from build123d import *

# Parameters (mm, degrees)
F0_R     = 4.1
F0_R_2   = 3.1
F1_DEPTH = 7
F2_SIZE  = 2


with BuildPart() as f1:
    # F0 (on Top) → F1 (new body)
    with BuildSketch(Plane.XY):
        with BuildLine():
            ThreePointArc((67.5, 27.5), (66.035534, 31.035534), (62.5, 32.5))
            Line((62.5, 32.5), (-62.5, 32.5))
            ThreePointArc((-62.5, 32.5), (-66.035534, 31.035534), (-67.5, 27.5))
            Line((-67.5, 27.5), (-67.5, -27.5))
            ThreePointArc((-67.5, -27.5), (-66.035534, -31.035534), (-62.5, -32.5))
            Line((-62.5, -32.5), (62.5, -32.5))
            ThreePointArc((62.5, -32.5), (66.035534, -31.035534), (67.5, -27.5))
            Line((67.5, -27.5), (67.5, 27.5))
        make_face()
        with Locations((-57, -23.5)):
            Circle(F0_R, mode=Mode.SUBTRACT)
        with Locations((0, -23.5)):
            Circle(F0_R_2, mode=Mode.SUBTRACT)
        with Locations((57, -23.5)):
            Circle(F0_R, mode=Mode.SUBTRACT)
        with Locations((-57, 23.5)):
            Circle(F0_R, mode=Mode.SUBTRACT)
        with BuildLine():
            Line((-31.75, 7.5), (31.75, 7.5))
            ThreePointArc((31.75, 7.5), (36.699747, 5.449747), (38.75, 0.5))
            Line((38.75, 0.5), (38.75, -0.5))
            ThreePointArc((38.75, -0.5), (36.699747, -5.449747), (31.75, -7.5))
            Line((31.75, -7.5), (-31.75, -7.5))
            ThreePointArc((-31.75, -7.5), (-36.699747, -5.449747), (-38.75, -0.5))
            Line((-38.75, -0.5), (-38.75, 0.5))
            ThreePointArc((-38.75, 0.5), (-36.699747, 5.449747), (-31.75, 7.5))
        make_face(mode=Mode.SUBTRACT)
        with Locations((0, 23.5)):
            Circle(F0_R_2, mode=Mode.SUBTRACT)
        with Locations((57, 23.5)):
            Circle(F0_R, mode=Mode.SUBTRACT)
    extrude(amount=F1_DEPTH)

    # F2
    f2_edges = [f1.edges().sort_by_distance(p)[0] for p in [
        (-52.9, -23.5, 3.5),
        (-61.1, -23.5, 0),
        (-61.1, -23.5, 7),
        (-52.9, 23.5, 3.5),
        (-61.1, 23.5, 0),
        (-61.1, 23.5, 7),
        (3.1, 23.5, 3.5),
        (-3.1, 23.5, 0),
        (-3.1, 23.5, 7),
        (61.1, 23.5, 3.5),
        (52.9, 23.5, 0),
        (52.9, 23.5, 7),
        (61.1, -23.5, 3.5),
        (52.9, -23.5, 0),
        (52.9, -23.5, 7),
        (3.1, -23.5, 3.5),
        (-3.1, -23.5, 0),
        (-3.1, -23.5, 7),
    ]]
    chamfer(f2_edges, length=F2_SIZE)


solid = f1.part
Verification items for the finished model (mm, model axes). A direction names the side the tool comes from. Round coordinates to 2 decimals unless told otherwise and drop trailing zeros. Loops run counter-clockwise (first coordinate to the right, second up) from the corner with the lowest first, then second, coordinate; pieces in that order, holes last. Notation, with made-up numbers: (79, 10) - (107, 10) arc R19 ccw to (107, 30) - close; hole circle Ø10 at (-31.75, 38). An arc over 180 degrees is marked (long way). Answer in a Markdown table with one row per item. Add a question column.
Q1. Section check A-A on x = 0. Enter the section's corners in (y, z).
Q2. Material ranges on line 1 (Y direction, x = -57, z = 3.15); line 2 (Y direction, x = 32, z = 3.5); line 3 (X direction, y = 25, z = 5.5), recorded low to high.
Q3. Section check B-B on x = -57. Enter the section's corners in (y, z).
Q4. Section check D-D on x = 21. Enter the section's corners in (y, z), plus the area to 3 significant figures.
Q5. Tool access check on faces 1 (the face through (0, -7.5, 3)), 2 (the face through (-57.916, 19.375, 1.875)). Record the directions out of +Z, -Z, +X, -X, +Y, -Y that give a thin tool (end or side, any length) a straight path to the whole face; none if there is none.
Q6. Release check for a two-part mould opening along Y. For faces 3 (the face through (1, 32.5, 3)), 4 (the face through (-57.916, 19.375, 5.125)), 5 (the face through (66, -31.07, 3.45)) record: pulls with the +Y half, pulls with the -Y half, needs draft (parallel to the pull), parting line crosses it, or undercut.
Q7. Section check C-C on y = -23.5. Enter the section's corners in (x, z), plus the area to 3 significant figures.
Q8. Gauge pin test, flat ends, axial feed: pin 1 (5 mm diameter, centred on x = -57, y = 23.5, fed in from +Z); pin 2 (9.5 mm diameter, centred on x = 57, y = -23.5, fed in from +Z); pin 3 (3 mm diameter, centred on x = -1, y = 25, fed in from -Z); pin 4 (10 mm diameter, centred on x = 0, y = -23.5, fed in from -Z). Record the tip position at first contact, or that the pin passes through.
Found:
| question | item | result |
|---|---|---|
| 1 | outline | (-32.5, 0) - (-28.6, 0) - (-26.6, 2) - (-26.6, 5) - (-28.6, 7) - (-32.5, 7) - close; (-20.4, 2) - (-18.4, 0) - (-7.5, 0) - (-7.5, 7) - (-18.4, 7) - (-20.4, 5) - close; (7.5, 0) - (18.4, 0) - (20.4, 2) - (20.4, 5) - (18.4, 7) - (7.5, 7) - close; (26.6, 2) - (28.6, 0) - (32.5, 0) - (32.5, 7) - (28.6, 7) - (26.6, 5) - close |
| 2 | line 1 | y = -32.5 to -27.6, -19.4 to 19.4, 27.6 to 32.5 |
| 2 | line 2 | y = -32.5 to -7.5, 7.5 to 32.5 |
| 2 | line 3 | x = -67.5 to -61.35, -52.65 to -3.27, 3.27 to 52.65, 61.35 to 67.5 |
| 3 | outline | (-32.5, 0) - (-29.6, 0) - (-27.6, 2) - (-27.6, 5) - (-29.6, 7) - (-32.5, 7) - close; (-19.4, 2) - (-17.4, 0) - (17.4, 0) - (19.4, 2) - (19.4, 5) - (17.4, 7) - (-17.4, 7) - (-19.4, 5) - close; (27.6, 2) - (29.6, 0) - (32.5, 0) - (32.5, 7) - (29.6, 7) - (27.6, 5) - close |
| 4 | outline | (-32.5, 0) - (-7.5, 0) - (-7.5, 7) - (-32.5, 7) - close; (7.5, 0) - (32.5, 0) - (32.5, 7) - (7.5, 7) - close |
| 4 | area | 350 mm² |
| 5 | face 1 | +Z, -Z |
| 5 | face 2 | -Z |
| 6 | face 3 | pulls with the +Y half |
| 6 | face 4 | undercut |
| 6 | face 5 | pulls with the -Y half |
| 7 | outline | (-67.5, 0) - (-63.1, 0) - (-61.1, 2) - (-61.1, 5) - (-63.1, 7) - (-67.5, 7) - close; (-52.9, 2) - (-50.9, 0) - (-5.1, 0) - (-3.1, 2) - (-3.1, 5) - (-5.1, 7) - (-50.9, 7) - (-52.9, 5) - close; (3.1, 2) - (5.1, 0) - (50.9, 0) - (52.9, 2) - (52.9, 5) - (50.9, 7) - (5.1, 7) - (3.1, 5) - close; (61.1, 2) - (63.1, 0) - (67.5, 0) - (67.5, 7) - (63.1, 7) - (61.1, 5) - close |
| 7 | area | 763 mm² |
| 8 | pin 1 | passes through |
| 8 | pin 2 | stops at z = 5.65 |
| 8 | pin 3 | stops at z = 1.8 |
| 8 | pin 4 | stops at z = 0.1 |
